```python
from build123d import *

# Parameters (mm, degrees)
PAD_DEPTH         = 15
SKETCH001_R       = 5
POCKET_DEPTH      = 35.001
POCKET_DEPTH_BACK = -14.001
SKETCH002_R       = 33.208943
SKETCH002_R_2     = 21.759288
POCKET001_DEPTH   = 49.001
CHAMFER_SIZE      = 1
CHAMFER001_SIZE   = 1
CHAMFER002_SIZE   = 1
CHAMFER003_SIZE   = 1
CHAMFER004_SIZE   = 1
CHAMFER005_SIZE   = 1


with BuildPart() as part:
    # Sketch → Pad (new body)
    with BuildSketch(Plane.XY):
        with BuildLine():
            ThreePointArc((0, 13.25), (-13.25, 0), (0, -13.25))
            Line((0, -20), (0, -13.25))
            Line((0, -20), (-44.732538, -20))
            ThreePointArc((-44.732538, 20), (-49, 0), (-44.732538, -20))
            Line((-44.732538, 20), (0, 20))
            Line((0, 13.25), (0, 20))
        make_face()
    extrude(amount=PAD_DEPTH)

    # Sketch001 → Pocket (cut, two sides)
    with BuildSketch(Plane.YZ.offset(-14)) as pocket_sk:
        with Locations((0, 7.5)):
            Circle(SKETCH001_R)
    extrude(amount=-POCKET_DEPTH, mode=Mode.SUBTRACT)
    extrude(pocket_sk.sketch, amount=-POCKET_DEPTH_BACK, mode=Mode.SUBTRACT)

    # Sketch002 → Pocket001 (cut, through all)
    with BuildSketch(Plane.YZ):
        with Locations((0, -6.869182)):
            Circle(SKETCH002_R)
        with Locations((0, -6.869182)):
            Circle(SKETCH002_R_2, mode=Mode.SUBTRACT)
    extrude(amount=-POCKET001_DEPTH, mode=Mode.SUBTRACT)

    # Chamfer
    chamfer_edges = [part.edges().sort_by_distance(p)[0] for p in [
        (-48.74423, -5, 7.5),
    ]]
    chamfer(chamfer_edges, length=CHAMFER_SIZE)

    # Chamfer001
    chamfer001_edges = [part.edges().sort_by_distance(p)[0] for p in [
        (-13.25, 0, 0),
    ]]
    chamfer(chamfer001_edges, length=CHAMFER001_SIZE)

    # Chamfer002
    chamfer002_edges = [part.edges().sort_by_distance(p)[0] for p in [
        (-49, 0, 14.890106),
    ]]
    chamfer(chamfer002_edges, length=CHAMFER002_SIZE)

    # Chamfer003
    chamfer003_edges = [part.edges().sort_by_distance(p)[0] for p in [
        (-13.25, 0, 14.890106),
    ]]
    chamfer(chamfer003_edges, length=CHAMFER003_SIZE)

    # Chamfer004
    chamfer004_edges = [part.edges().sort_by_distance(p)[0] for p in [
        (0, -17.48534, 6.081861),
    ]]
    chamfer(chamfer004_edges, length=CHAMFER004_SIZE)

    # Chamfer005
    chamfer005_edges = [part.edges().sort_by_distance(p)[0] for p in [
        (0, 17.485451, 6.081711),
    ]]
    chamfer(chamfer005_edges, length=CHAMFER005_SIZE)


solid = part.part
```
Input: part model. Units: mm. Frame: model coordinates. Give positions to 0.01 mm unless a question says otherwise; leave off trailing zeros. Loops run counter-clockwise (first coordinate to the right, second up) from the corner with the lowest first, then second, coordinate; pieces in that order, holes last.
1) Contact query for flat-ended pins moving along their axis: pin 1 (4 mm diameter, centred on y = 9.5, z = 3, fed in from +X); pin 2 (2 mm diameter, centred on x = -37.5, y = -10.5, fed in from -Z); pin 3 (1 mm diameter, centred on x = -7, z = 9.5, fed in from -Y); pin 4 (1.5 mm diameter, centred on y = -8.5, z = 3.5, fed in from -X). Output: stop coordinate, or through.
A:
pin 1: stops at x = -6.58
pin 2: stops at z = 0
pin 3: stops at y = -14.89
pin 4: stops at x = -48.38
2) Mould query, pull axis Y, two halves, no side actions, for faces 1 (the flat face through (-22, -20, 1)), 2 (the cylindrical face through (-12.35, 4.8, 4.49)), 3 (the flat face through (0, 16, 3)). Classes: released by +Y, released by -Y, zero draft, split by the parting line, or undercut.
A:
face 1: released by -Y
face 2: undercut
face 3: zero draft
3) Section query A-A on x = -33. Return the cut outline in (y, z).
A:
outline: (-20, 0) - (20, 0) - (20, 1.7) arc R21.76 ccw to (-20, 1.7) - close; hole circle Ø10 at (0, 7.5)
4) Line query: L1, parallel to Z at x = -22, y = 0; L2, parallel to Y at x = -39, z = 11.25; L3, parallel to Y at x = -10, z = 3.5. Output: solid intervals per line, ascending.
A:
L1: z = 0 to 2.5, 12.5 to 14.89
L2: y = -12.05 to -3.31, 3.31 to 12.05
L3: y = -19.13 to -8.69, 8.69 to 19.13
